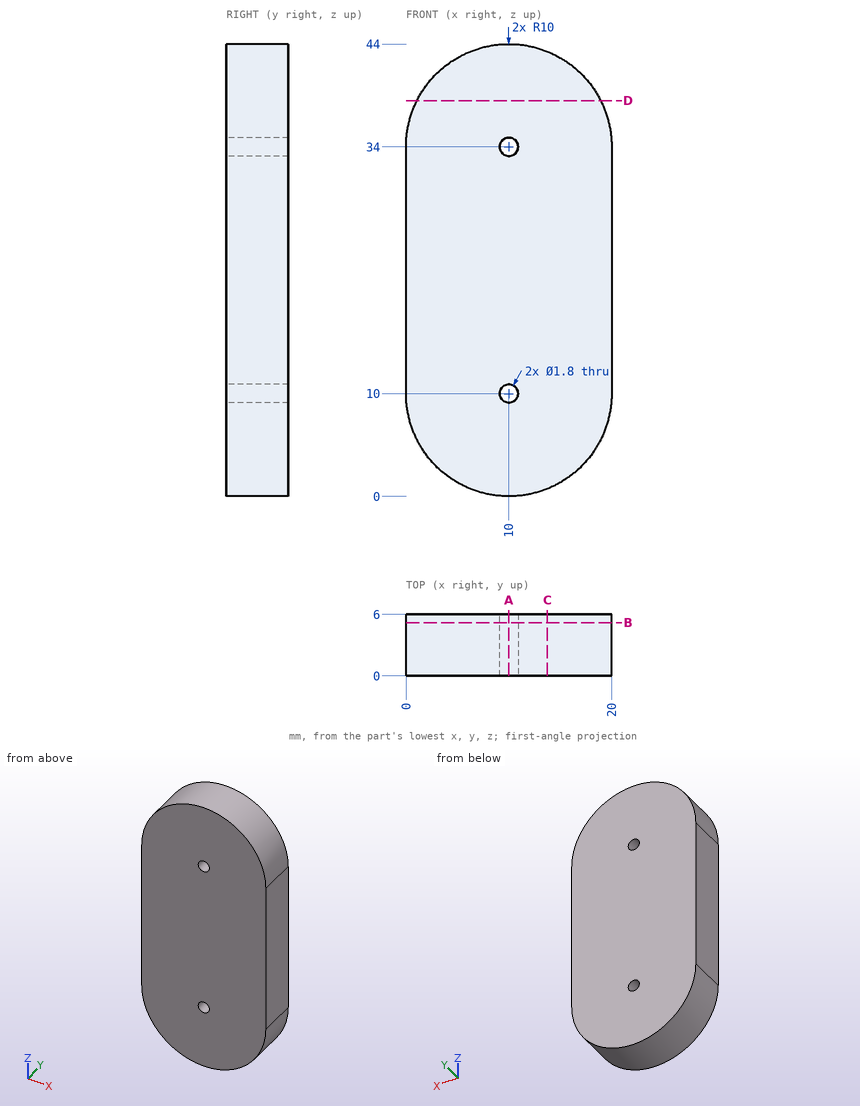
For this review, use the dimensioned drawing (mm, ordinates from the lowest corner) and the shaded views. Coordinates: 2 decimals unless noted, no trailing zeros. Order: outer loops, then holes, each group sorted by start corner. A loop starts at its lowest first (then second) coordinate and runs counter-clockwise, first axis right, second up. Notation, with made-up numbers: (-25, -29.75) - (10, -29.75) arc R12 ccw to (10, -14.75) - close; hole circle Ø9 at (-11.5, 68). An arc over 180 degrees is marked (long way). Use one line per item in the form item = value.
Q1. Consider section A-A (x = 10). Give the boundary of the cut face in (y, z), then the cut area to 3 significant figures.
Checked values:
outline = (0, 0) - (6, 0) - (6, 9.1) - (0, 9.1) - close; (0, 10.9) - (6, 10.9) - (6, 33.1) - (0, 33.1) - close; (0, 34.9) - (6, 34.9) - (6, 44) - (0, 44) - close
area = 242 mm2
Q2. Consider section C-C (x = 13.75). Give the boundary of the cut face in (y, z), then the cut area to 3 significant figures.
Checked values:
outline = (0, 0.73) - (6, 0.73) - (6, 43.27) - (0, 43.27) - close
area = 255 mm2
Q3. For probe 1 along Z at (x, y) = (10, 1.9); probe 2 along X at (y, z) = (4.75, 34); probe 3 along Z at (x, y) = (9.5, 2.55), list the stretches that pass through material, from the lowest coordinate up. Write a range as from..to.
Checked values:
probe_1 = 0..9.1, 10.9..33.1, 34.9..44
probe_2 = 0..9.1, 10.9..20
probe_3 = 0.01..9.25, 10.75..33.25, 34.75..43.99
Q4. Consider section D-D (z = 38.5). Give the boundary of the cut face in (x, y).
Checked values:
outline = (1.07, 0) - (18.93, 0) - (18.93, 6) - (1.07, 6) - close
Q5. Consider section B-B (y = 5.2). Give the boundary of the cut face in (x, z), then the cut area to 3 significant figures.
Checked values:
outline = (0, 10) arc R10 ccw to (20, 10) - (20, 34) arc R10 ccw to (0, 34) - close; hole circle Ø1.8 at (10, 10); hole circle Ø1.8 at (10, 34)
area = 789 mm2
Q6. For P1, Ø1.6, axis at x = 10, z = 34, coming from the +Y side, flat-tipped, find the tip position at first contact; note if it passes through.
Checked values:
P1 = through
